Can you work these out from the model? Positions are in its coordinate system, mm. A direction names the side the tool comes from. Give positions to 0.01 mm unless a question says otherwise; leave off trailing zeros. Loops run counter-clockwise (first coordinate to the right, second up) from the corner with the lowest first, then second, coordinate; pieces in that order, holes last. Notation, with made-up numbers: M 77.25,-5 L 127.25,-5 A20 ccw 127.25,24 Z; hole C 58.25,39.5 d5. An arc over 180 degrees is marked long. Use CSV: the item, a comma, the result in double quotes.
Autodesk Inventor part; units mm, degrees
ref_plane "YZ Plane" through (0, 0, 0) normal (1, 0, 0) x (0, 1, 0)
ref_plane "XZ Plane" through (0, 0, 0) normal (0, 1, 0) x (-1, 0, 0)
ref_plane "XY Plane" through (0, 0, 0) normal (0, 0, 1) x (1, 0, 0)
sketch "Sketch1" plane through (0, 0, 0) normal (1, 0, 0) x (0, 1, 0)
  line L0 (0, 0) -> (-3, 0)
  line L1 (0, 28.5) -> (0, 33)
  line L2 (0, 33) -> (-1, 33)
  line L3 (-1, 33) -> (-1, 29.5)
  line L4 (-1, 29.5) -> (-3, 29.5)
  line L5 (-3, 29.5) -> (-3, 0)
  line L6 (0, 28.5) -> (-1, 28.5)
  line L7 (-1, 28.5) -> (-1, 5)
  line L8 (-2, 2.5) -> (-3, 2.5)
  line L9 (-1, 5) -> (-2, 5)
  line L10 (-2, 5) -> (-2, 0)
  line L11 (0, 33) -> (0, 0) construction
  line L12 (-1, 5) -> (0, 5)
  line L13 (-1, 6) -> (0, 6)
  line L14 (0, 5) -> (0, 6)
  line L15 (0, 6) -> (0, 0)
  line L16 (0, 0) -> (-3, 0)
  point P0 (-1, 2.5)
  point P1 (0, 5)
  dimension "d0" = 66
  dimension "d2" = 3
  dimension "d3" = 1
  dimension "d6" = 1
  dimension "d20" = 5
  dimension "d21" = 10
  dimension "d22" = 1
  dimension "d23" = 1
  dimension "d31" = 59
  dimension "d32" = 1
revolve "Revolution1" add sketch "Sketch1" angle 360 about axis through (0, 0, 0) along (0, -1, 0)
sketch "Sketch2" plane through (0, -1, 0) normal (0, 1, 0) x (1, 0, 0)
  arc A0 (-24.6817, 14.25) -> (-24.6817, -14.25) centre (0, 0) ccw
  line L0 (-1.7321, -1) -> (-24.6817, -14.25)
  line L1 (-1.7321, 1) -> (-24.6817, 14.25)
  arc A1 (-1.7321, 1) -> (-1.7321, -1) centre (0, 0) ccw
  line L2 (-28.5, 0) -> (0, 0) construction
  line L3 (0, 0) -> (-24.6817, -14.25) construction
  line L4 (0, 0) -> (-24.6817, 14.25) construction
  line L5 (-21.8856, -8.0169) -> (-9.5, -0.866)
  arc A2 (-5.873, -1.228) -> (-5.873, 1.228) centre (0, 0) ccw
  line L6 (-9.5, 0.866) -> (-21.8856, 8.0169)
  arc A3 (-23.3382, 7.4551) -> (-23.3382, -7.4551) centre (0, 0) ccw
  arc A4 (-9.5, -0.866) -> (-9.5, 0.866) centre (-10, 0) ccw
  arc A5 (-21.8856, 8.0169) -> (-23.3382, 7.4551) centre (-22.3856, 7.1508) ccw
  arc A6 (-23.3382, -7.4551) -> (-21.8856, -8.0169) centre (-22.3856, -7.1508) ccw
  arc A7 (-18.1254, -16.4839) -> (-5.2128, -23.939) centre (0, 0) ccw
  arc A8 (-5.2128, -23.939) -> (-4, -22.9619) centre (-5, -22.9619) ccw
  line L7 (-4, -22.9619) -> (-4, -8.6603)
  arc A9 (-4, -8.6603) -> (-5.5, -7.7942) centre (-5, -8.6603) ccw
  line L8 (-5.5, -7.7942) -> (-17.8856, -14.9451)
  arc A10 (-17.8856, -14.9451) -> (-18.1254, -16.4839) centre (-17.3856, -15.8111) ccw
  arc A11 (5.2128, -23.939) -> (18.1254, -16.4839) centre (0, 0) ccw
  arc A12 (18.1254, -16.4839) -> (17.8856, -14.9451) centre (17.3856, -15.8111) ccw
  line L9 (17.8856, -14.9451) -> (5.5, -7.7942)
  arc A13 (5.5, -7.7942) -> (4, -8.6603) centre (5, -8.6603) ccw
  line L10 (4, -8.6603) -> (4, -22.9619)
  arc A14 (4, -22.9619) -> (5.2128, -23.939) centre (5, -22.9619) ccw
  arc A15 (23.3382, -7.4551) -> (23.3382, 7.4551) centre (0, 0) ccw
  arc A16 (23.3382, 7.4551) -> (21.8856, 8.0169) centre (22.3856, 7.1508) ccw
  line L11 (21.8856, 8.0169) -> (9.5, 0.866)
  arc A17 (9.5, 0.866) -> (9.5, -0.866) centre (10, 0) ccw
  line L12 (9.5, -0.866) -> (21.8856, -8.0169)
  arc A18 (21.8856, -8.0169) -> (23.3382, -7.4551) centre (22.3856, -7.1508) ccw
  arc A19 (18.1254, 16.4839) -> (5.2128, 23.939) centre (0, 0) ccw
  arc A20 (5.2128, 23.939) -> (4, 22.9619) centre (5, 22.9619) ccw
  line L13 (4, 22.9619) -> (4, 8.6603)
  arc A21 (4, 8.6603) -> (5.5, 7.7942) centre (5, 8.6603) ccw
  line L14 (5.5, 7.7942) -> (17.8856, 14.9451)
  arc A22 (17.8856, 14.9451) -> (18.1254, 16.4839) centre (17.3856, 15.8111) ccw
  arc A23 (-5.2128, 23.939) -> (-18.1254, 16.4839) centre (0, 0) ccw
  arc A24 (-18.1254, 16.4839) -> (-17.8856, 14.9451) centre (-17.3856, 15.8111) ccw
  line L15 (-17.8856, 14.9451) -> (-5.5, 7.7942)
  arc A25 (-5.5, 7.7942) -> (-4, 8.6603) centre (-5, 8.6603) ccw
  line L16 (-4, 8.6603) -> (-4, 22.9619)
  arc A26 (-4, 22.9619) -> (-5.2128, 23.939) centre (-5, 22.9619) ccw
  circle A27 centre (0, 0) radius 28.5 construction
  point P0 (-22.9329, -8.6215)
  point P1 (-22.9329, 8.6215)
  point P2 (-4, -4.4721)
  point P3 (-1.873, -5.7002)
  point P4 (1.873, -5.7002)
  point P5 (4, -4.4721)
  point P6 (5.873, -1.228)
  point P7 (5.873, 1.228)
  point P8 (4, 4.4721)
  point P9 (1.873, 5.7002)
  point P10 (-1.873, 5.7002)
  point P11 (-4, 4.4721)
  dimension "d7" = 60
  dimension "d8" = 2
  dimension "d13" = 4
  dimension "d15" = 1
  dimension "d18" = 360
extrude "Extrusion1" cut sketch "Sketch2" against normal through all contours A6 A3 A5 L6 A4 L5 | A10 L8 A9 L7 A8 A7 | A14 L10 A13 L9 A12 A11 | A18 L12 A17 L11 A16 A15 | A22 L14 A21 L13 A20 A19 | A26 L16 A25 L15 A24 A23
sketch "Sketch3" plane through (0, 0, 0) normal (0, 1, 0) x (1, 0, 0)
  line L0 (3.5, -2) -> (-3.5, -2)
  line L1 (-3.5, -2) -> (-3.5, 2)
  line L2 (-3.5, 2) -> (3.5, 2)
  line L3 (3.5, 2) -> (3.5, -2)
  line L4 (3.5, -2) -> (-3.5, 2) construction
  line L5 (-3.5, -2) -> (3.5, 2) construction
  circle A0 centre (0, 0) radius 33
  circle A1 centre (0, 0) radius 28.5
  circle A2 centre (0, 0) radius 6
  line L6 (-5.6569, -2) -> (5.6569, -2)
  circle A3 centre (0, 0) radius 6
  line L7 (-5.6569, 2) -> (5.6569, 2)
  line L8 (-4.5, -2) -> (-4.5, 2)
  line L9 (4.5, 2) -> (4.5, -2)
  line L10 (0, -2) -> (0, 2) construction
  point P0 (3.5, 2)
  point P1 (3.5, -2)
  point P2 (-3.5, -2)
  point P3 (-3.5, 2)
  dimension "d24" = 4
  dimension "d27" = 9
  dimension "d36" = 7
extrude "Extrusion2" cut sketch "Sketch3" against normal through all contours L0 L1 L2 L3
extrude "Extrusion3" cut sketch "Sketch3" against normal blind 2 contours L3 L7 L9 L6 | L6 L8 L7 L1
chamfer "Chamfer1" distance 1 angle 45 2 edges at (-4.5, -2, 0) (4.5, -2, 0)
sketch "Sketch4" plane through (0, -3, 0) normal (0, -1, 0) x (1, 0, 0)
  line L0 (-3.5, -2) -> (3.5, -2)
  line L1 (3.5, -2) -> (3.5, 2)
  line L2 (3.5, 2) -> (-3.5, 2)
  line L3 (-3.5, 2) -> (-3.5, -2)
  arc A0 (18.1254, -16.4839) -> (17.8856, -14.9451) centre (17.3856, -15.8111) ccw
  line L4 (17.8856, -14.9451) -> (5.5, -7.7942)
  arc A1 (5.5, -7.7942) -> (4, -8.6603) centre (5, -8.6603) ccw
  line L5 (4, -8.6603) -> (4, -22.9619)
  arc A2 (4, -22.9619) -> (5.2128, -23.939) centre (5, -22.9619) ccw
  arc A3 (5.2128, -23.939) -> (18.1254, -16.4839) centre (0, 0) ccw
  arc A4 (-18.1254, 16.4839) -> (-17.8856, 14.9451) centre (-17.3856, 15.8111) ccw
  line L6 (-17.8856, 14.9451) -> (-5.5, 7.7942)
  arc A5 (-5.5, 7.7942) -> (-4, 8.6603) centre (-5, 8.6603) ccw
  line L7 (-4, 8.6603) -> (-4, 22.9619)
  arc A6 (-4, 22.9619) -> (-5.2128, 23.939) centre (-5, 22.9619) ccw
  arc A7 (-5.2128, 23.939) -> (-18.1254, 16.4839) centre (0, 0) ccw
  arc A8 (-5.2128, -23.939) -> (-4, -22.9619) centre (-5, -22.9619) ccw
  line L8 (-4, -22.9619) -> (-4, -8.6603)
  arc A9 (-4, -8.6603) -> (-5.5, -7.7942) centre (-5, -8.6603) ccw
  line L9 (-5.5, -7.7942) -> (-17.8856, -14.9451)
  arc A10 (-17.8856, -14.9451) -> (-18.1254, -16.4839) centre (-17.3856, -15.8111) ccw
  arc A11 (-18.1254, -16.4839) -> (-5.2128, -23.939) centre (0, 0) ccw
  arc A12 (23.3382, 7.4551) -> (21.8856, 8.0169) centre (22.3856, 7.1508) ccw
  line L10 (21.8856, 8.0169) -> (9.5, 0.866)
  arc A13 (9.5, 0.866) -> (9.5, -0.866) centre (10, 0) ccw
  line L11 (9.5, -0.866) -> (21.8856, -8.0169)
  arc A14 (21.8856, -8.0169) -> (23.3382, -7.4551) centre (22.3856, -7.1508) ccw
  arc A15 (23.3382, -7.4551) -> (23.3382, 7.4551) centre (0, 0) ccw
  arc A16 (5.2128, 23.939) -> (4, 22.9619) centre (5, 22.9619) ccw
  line L12 (4, 22.9619) -> (4, 8.6603)
  arc A17 (4, 8.6603) -> (5.5, 7.7942) centre (5, 8.6603) ccw
  line L13 (5.5, 7.7942) -> (17.8856, 14.9451)
  arc A18 (17.8856, 14.9451) -> (18.1254, 16.4839) centre (17.3856, 15.8111) ccw
  arc A19 (18.1254, 16.4839) -> (5.2128, 23.939) centre (0, 0) ccw
  arc A20 (-21.8856, 8.0169) -> (-23.3382, 7.4551) centre (-22.3856, 7.1508) ccw
  arc A21 (-23.3382, 7.4551) -> (-23.3382, -7.4551) centre (0, 0) ccw
  arc A22 (-23.3382, -7.4551) -> (-21.8856, -8.0169) centre (-22.3856, -7.1508) ccw
  line L14 (-21.8856, -8.0169) -> (-9.5, -0.866)
  arc A23 (-9.5, -0.866) -> (-9.5, 0.866) centre (-10, 0) ccw
  line L15 (-9.5, 0.866) -> (-21.8856, 8.0169)
  circle A24 centre (0, 0) radius 29.5
  circle A25 centre (0, 0) radius 15
  dimension "d33" = 30
extrude "Extrusion4" add sketch "Sketch4" against normal blind 1 contours A25 L5 A1 L4 | L4 A1 L5 A25 L8 A9 L9 L14 A23 L15 L6 A5 L7 L12 A17 L13 L10 A13 L11 | L11 A13 L10 A25 | A25 L9 A9 L8 | A25 L15 A23 L14 | L13 A17 L12 A25 | A25 L7 A5 L6
fillet "Fillet2" radius 1 12 edges at (4, -2.5, -14.4568) (10.52, -2.5, -10.6925) (14.52, -2.5, -3.7643) (14.52, -2.5, 3.7643) (10.52, -2.5, 10.6925) (4, -2.5, 14.4568) (-4, -2.5, 14.4568) (-14.52, -2.5, -3.7643) (-4, -2.5, -14.4568) (-10.52, -2.5, -10.6925) (-14.52, -2.5, 3.7643) (-10.52, -2.5, 10.6925)
properties part number "FS-03-SLBV1"
Q1. I want a section at A-A, the plane x = 0. Please give me the cut outline in (y, z).
Model answer:
outline,"M -3,-29.5 L -1,-29.5 L -1,-33 L 0,-33 L 0,-28.5 L -1,-28.5 L -1,-6 L 0,-6 L 0,-2 L -3,-2 Z; M -3,2 L 0,2 L 0,6 L -1,6 L -1,28.5 L 0,28.5 L 0,33 L -1,33 L -1,29.5 L -3,29.5 Z"
Q2. For faces 3 (the flat face through (17.16, -1.76, -5.29)), 4 (the cylindrical face through (7.463, -2.507, -13.012)), which set-ups out of +Z, -Z, +X, -X, +Y, -Y let a thin tool reach every point of the face, with its end or its side?
Model answer:
face 3,"+Y"
face 4,"+Y, -Y"
Q3. I want a section at B-B, the plane z = -5. Please give me the cut outline in (x, y).
Model answer:
outline,"M -32.62,-1 L -29.07,-1 L -29.07,-3 L -23.98,-3 L -23.98,-1 L -28.06,-1 L -28.06,0 L -32.62,0 Z; M -16.66,-3 L 16.66,-3 L 16.66,-1 L 3.32,-1 L 3.32,0 L -3.32,0 L -3.32,-1 L -16.66,-1 Z; M 23.98,-3 L 29.07,-3 L 29.07,-1 L 32.62,-1 L 32.62,0 L 28.06,0 L 28.06,-1 L 23.98,-1 Z"
Q4. I want a section at C-C, the plane z = 25.5. Please give me the cut outline in (x, y).
Model answer:
outline,"M -20.95,-1 L -14.83,-1 L -14.83,-3 L 14.83,-3 L 14.83,-1 L 20.95,-1 L 20.95,0 L 12.73,0 L 12.73,-1 L -12.73,-1 L -12.73,0 L -20.95,0 Z"
Q5. If we mould it in two halves opening along Z, with no side actions, what happens to faces 1 (the flat face through (13, -2, 0)), 2 (the cylindrical face through (10.916, -0.507, 26.327))? For each: released by +Z, released by -Z, zero draft, split by the parting line, or undercut.
Model answer:
face 1,"undercut"
face 2,"undercut"
Q6. Please list where these lines run through material, in increasing order: L1, parallel to Z at x = 0, y = -0.4; L2, parallel to X at y = -0.3, z = 0; L3, parallel to Z at x = -16, y = -1.65. Write a range as from..to.
Model answer:
L1,"-33..-28.5, -6..-2, 2..6, 28.5..33"
L2,"-33..-28.5, -6..-4.5, 4.5..6, 28.5..33"
L3,"-24.78..-18.55, -13.86..-4.62, 4.62..13.86, 18.55..24.78"
Q7. I want a section at D-D, the plane x = 20.5. Please give me the cut outline in (y, z), then the cut area to 3 significant figures.
Model answer:
outline,"M -3,-21.21 L -1,-21.21 L -1,-25.86 L 0,-25.86 L 0,-19.8 L -1,-19.8 L -1,-7.22 L -3,-7.22 Z; M -3,7.22 L -1,7.22 L -1,19.8 L 0,19.8 L 0,25.86 L -1,25.86 L -1,21.21 L -3,21.21 Z"
area,"68.1 mm2"
Q8. I'm going to push flat-ended pins straight in: P1, Ø0.5, axis at y = -2.5, z = 0, coming from the +X side; P2, Ø1.8, axis at x = 13, z = -1.5, coming from the +Y side; P3, Ø1, axis at x = -24.5, y = -2, coming from the +Z side. Where does each tip first touch, or does it pass through?
Model answer:
P1,"x = 29.5"
P2,"y = -2"
P3,"z = 17.15"
